Design review of the part built by this model. Coordinates are the model's own, in mm. A direction names the side the tool comes from. Round coordinates to 2 decimals unless told otherwise and drop trailing zeros. Loops run counter-clockwise (first coordinate to the right, second up) from the corner with the lowest first, then second, coordinate; pieces in that order, holes last. Notation, with made-up numbers: M 30.25,75 L 62.25,75 A20 ccw 62.25,91 Z; hole C 40,-21 d4. An arc over 180 degrees is marked long. One line per item, written item: value. Start each with the question number.
Item 1: We need section B-B (z = 24). State how many separate pieces and enclosed holes the cut face has, then the cut area to 3 significant figures.
Item 2: For line 1 along X through (y, z) = (-4, 18); line 2 along Y through (x, z) = (6.5, 12.5); line 3 along X through (y, z) = (-17, 28), list the stretches that pass through material, from the lowest coordinate up.
Item 3: We need section C-C (x = 15). Write out the cut boundary in (y, z) (3 decimals), then the cut area to 3 significant figures.
Item 4: We need section A-A (z = 20). Write out the cut boundary in (x, y).
Item 5: For faces 1 (the flat face through (28.151, -6.994, 35.993)), 2 (the flat face through (5.06, -15.83, 7.83)), 3 (the flat face through (14, -32.4, 15.8)), 4 (the flat face through (13, -22.86, 19)), 5 (the flat face through (22.2, -4.7, 30.1)), list the 3-axis set-ups (+Z, -Z, +X, -X, +Y, -Y) from which the entire face can be reached by the end or side of a thin tool; tool diameter is ignored.
Item 6: Clearance check with flat-ended pins moving along their axes: pin 1 (1.5 mm diameter, centred on x = 30, y = -18, fed in from +Z) (3 decimals); pin 2 (6 mm diameter, centred on y = -11, z = 27, fed in from +X); pin 3 (5 mm diameter, centred on x = 31.5, z = 11.5, fed in from -Y); pin 4 (2 mm diameter, centred on x = 17, z = 31, fed in from +Y). State where each tip first meets the part, or that it passes through.
Item 7: Mouldability with a two-part tool opening along X and no side actions: class faces 6 (the flat face through (15.83, -33.5, 30.27)), 7 (the flat face through (12.7, -10.6, 23.3)), 8 (the flat face through (33.2, -22.2, 8)) as released by +X, released by -X, zero draft, split by the parting line, or undercut.
from build123d import *

# Parameters (mm, degrees)
F0_W      = 38.1
F0_H      = 38.1
F1_DEPTH  = 38.1
F6_DEPTH  = 38.1
F8_DEPTH  = 38.1
F9_W      = 25.4
F9_H      = 7.62
F10_DEPTH = 38.1


with BuildPart() as f1:
    # F0 (on Front) → F1 (new body)
    with BuildSketch(Plane.XZ):
        with Locations((19.05, 19.05)):
            Rectangle(F0_W, F0_H)
    extrude(amount=F1_DEPTH)

    # F5 (on offset) → F6 (cut)
    with BuildSketch(Plane.YZ.offset(38.1)):
        Polygon((-11.43, 21.477904), (-6.35, 38.1), (-31.750008, 38.1), (-26.67, 21.477904), (-21.59, 28.575), (-16.51, 28.575), align=None)
        Polygon((-31.750008, 0), (-38.100008, 38.1), (-38.100008, 0), align=None)
        Polygon((-25.400008, 0), (-12.700008, 0), (-19.050008, 15.875), align=None)
        Polygon((-6.35, 0), (0, 0), (0, 38.1), align=None)
    extrude(amount=-F6_DEPTH, mode=Mode.SUBTRACT)

    # F7 (on offset) → F8 (cut)
    with BuildSketch(Plane.XZ.offset(38.1)):
        Polygon((11.43, 22.225), (6.35, 0), (31.75, 0), (26.67, 22.225), (21.59, 9.525), (16.51, 9.525), align=None)
        Polygon((0, 0), (6.35, 38.1), (0, 38.1), align=None)
        Polygon((25.4, 38.1), (12.7, 38.1), (19.05, 22.225), align=None)
        Polygon((38.1, 38.1), (31.75, 38.1), (38.1, 0), align=None)
    extrude(amount=-F8_DEPTH, mode=Mode.SUBTRACT)

    # F9 (on offset) → F10 (cut)
    with BuildSketch(Plane.XY.offset(38.1)):
        with Locations((25.4, -11.43)):
            Rectangle(F9_W, F9_H)
        with Locations((12.7, -26.67)):
            Rectangle(F9_W, F9_H)
    extrude(amount=-F10_DEPTH, mode=Mode.SUBTRACT)


solid = f1.part
A:
1. separate pieces: 6
1. enclosed holes: 0
1. area: 609 mm2
2. line 1: 3 to 10.46, 13.12 to 24.98, 27.64 to 35.1
2. line 2: -33.83 to -30.48, -22.86 to -20.4, -17.7 to -4.27
2. line 3: 4.67 to 16.74, 21.36 to 33.43
3. outline: M -37.142,32.35 L -33.967,13.3 L -30.48,13.3 L -30.48,32.35 Z; M -22.86,13.3 L -20.08,13.3 L -19.05,15.875 L -18.02,13.3 L -15.24,13.3 L -15.24,26.801 L -16.51,28.575 L -21.59,28.575 L -22.86,26.801 Z; M -7.62,13.3 L -4.133,13.3 L -0.958,32.35 L -7.62,32.35 Z
3. area: 305 mm2
4. outline: M 3.33,-35.08 L 10.92,-35.08 L 10.92,-30.48 L 3.33,-30.48 Z; M 3.33,-22.86 L 10.92,-22.86 L 10.92,-3.02 L 3.33,-3.02 Z; M 12.32,-35.08 L 25.78,-35.08 L 25.78,-15.24 L 12.7,-15.24 L 12.7,-7.62 L 25.78,-7.62 L 25.78,-3.02 L 12.32,-3.02 L 12.32,-22.86 L 25.4,-22.86 L 25.4,-30.48 L 12.32,-30.48 Z; M 27.18,-35.08 L 34.77,-35.08 L 34.77,-15.24 L 27.18,-15.24 Z; M 27.18,-7.62 L 34.77,-7.62 L 34.77,-3.02 L 27.18,-3.02 Z
5. face 1: +Z, +X, -X
5. face 2: -Z, +X, -X
5. face 3: -Z, +Y, -Y
5. face 4: +Z, -Z, -X
5. face 5: +Z, +Y, -Y
6. pin 1: z = 28.575
6. pin 2: x = 12.7
6. pin 3: y = -34.08
6. pin 4: through
7. face 6: undercut
7. face 7: released by +X
7. face 8: zero draft
